```python
from build123d import *

# Parameters (mm, degrees)
PAD_DEPTH       = 20
SKETCH001_W     = 55
SKETCH001_H     = 5
PAD001_DEPTH    = 37
SKETCH002_W     = 8
SKETCH002_H     = 37
PAD002_DEPTH    = 2
SKETCH003_R     = 3.1
POCKET_DEPTH    = 7.001
CHAMFER_SIZE    = 7
FILLET_R        = 2
CHAMFER001_SIZE = 1


with BuildPart() as part:
    # Sketch → Pad (new body)
    with BuildSketch(Plane.XY):
        Polygon((-31.15, 0), (31.15, 0), (31.15, 31.5), (28.15, 31.5), (28.15, 34.5), (34.15, 34.5), (34.15, -3.5), (17.35, -25), (17.35, -33), (-29.15, -33), (-29.15, -11), (-34.15, -3.5), (-34.15, 34.5), (-28.15, 34.5), (-28.15, 31.5), (-31.15, 31.5), align=None)
        Polygon((-21.15, -8), (20.481035, -8), (7.197314, -25), (-21.15, -25), align=None, mode=Mode.SUBTRACT)
    extrude(amount=PAD_DEPTH)

    # Sketch001 (on Face21 of Pad) → Pad001 (join)
    with BuildSketch(Plane(origin=(0, 0, 0), x_dir=(1, 0, 0), z_dir=(0, 0, -1))):
        with Locations((-10.15, 30.5)):
            Rectangle(SKETCH001_W, SKETCH001_H)
    extrude(amount=-PAD001_DEPTH)

    # Sketch002 (on Face25 of Pad001) → Pad002 (join)
    with BuildSketch(Plane.XZ.offset(33)):
        with Locations((4.55, 18.5)):
            Rectangle(SKETCH002_W, SKETCH002_H)
        with Locations((-25.45, 18.5)):
            Rectangle(SKETCH002_W, SKETCH002_H)
    extrude(amount=PAD002_DEPTH)

    # Sketch003 (on Face19 of Pad002) → Pocket (cut, through all)
    with BuildSketch(Plane(origin=(0, -28, 0), x_dir=(-1, 0, 0), z_dir=(0, 1, 0))):
        with Locations((-4.55, 27)):
            Circle(SKETCH003_R)
        with Locations((25.45, 27)):
            Circle(SKETCH003_R)
    extrude(amount=-POCKET_DEPTH, mode=Mode.SUBTRACT)

    # Chamfer
    chamfer_edges = [part.edges().sort_by_distance(p)[0] for p in [
        (-37.65, -30.5, 37),
        (17.35, -30.5, 37),
    ]]
    chamfer(chamfer_edges, length=CHAMFER_SIZE)

    # Fillet
    fillet_edges = [part.edges().sort_by_distance(p)[0] for p in [
        (-29.15, -28, 10),
        (-29.15, -11, 10),
        (-34.15, -3.5, 10),
        (17.35, -25, 10),
        (34.15, -3.5, 10),
        (7.197314, -25, 10),
        (20.481035, -8, 10),
        (-21.15, -8, 10),
        (-21.15, -25, 10),
    ]]
    fillet(fillet_edges, radius=FILLET_R)

    # Chamfer001
    chamfer001_edges = [part.edges().sort_by_distance(p)[0] for p in [
        (-34.15, -28, 33.5),
        (-37.65, -28, 15),
        (-10.15, -28, 37),
        (13.85, -28, 33.5),
        (17.35, -28, 25),
    ]]
    chamfer(chamfer001_edges, length=CHAMFER001_SIZE)


solid = part.part
```
Part model, mm, in its own coordinate system. A direction names the side the tool comes from. Round coordinates to 2 decimals unless told otherwise and drop trailing zeros. Write each loop counter-clockwise with the first axis right and the second up, starting at its lowest first coordinate (ties: lowest second). Pieces come first, ordered by that corner, then holes. Notation, with made-up numbers: (39, 10) -> (89, 10) arc R24 cw to (89, 24) -> close; hole circle Ø3 at (-1.5, 14). An arc over 180 degrees is marked (long way). Return JSON: item names as keys, results as strings. Group by question number.
Q1. Which spindle directions (+Z, -Z, +X, -X, +Y, -Y) get a long thin tool onto all of the face, cutting with end or side? Do faces 4 (the flat face through (-21.45, -34, 18)), 5 (the flat face through (-31.62, -7.295, 9.86)), 6 (the flat face through (-16, -28, 26)). Say none if no direction does.
Q2. Pin check, flat tips, straight feed: pin 1 (1.5 mm diameter, centred on x = 22.5, y = -11.5, fed in from +Z); pin 2 (8 mm diameter, centred on y = -28, z = 19.5, fed in from +X); pin 3 (5 mm diameter, centred on y = -14, z = 21.5, fed in from -X). Stop position of each tip, or through.
Q3. Mould opens along Z. For faces 1 (the cylindrical face through (-27.12, -31.45, 29.61)), 2 (the flat face through (13.9, -30.97, 33.45)), 3 (the flat face through (-31.15, 16, 10)) say: pulls with the +Z half, pulls with the -Z half, needs draft (parallel to the pull), parting line crosses it, or undercut.
Q4. Saw through at B-B on z = 27. Write the cut outline in (x, y), plus the area to 3 significant figures.
Q5. Saw through at C-C on x = 4.55. Write the cut outline in (y, z).
Q6. Saw through at A-A on x = -25.45. Write the cut outline in (y, z), plus the area to 3 significant figures.
Q7. Probe L1, parallel to Y at x = 4, z = 11; L2, parallel to Z at x = 4.55, y = -32.25; L3, parallel to X at y = 14, z = 4.5. List the from-to ranges inside material, lowest first. Write a range as [from, to].
Q8. Saw through at D-D on y = -22. Write the cut outline in (x, z).
Answer:
{
 "1": {"face 4": "+Z, -Z, -Y", "face 5": "+Z, -Z, -X", "face 6": "+Z, -X"},
 "2": {"pin 1": "z = 20", "pin 2": "x = 18.13", "pin 3": "x = -29.15"},
 "3": {"face 1": "undercut", "face 2": "pulls with the +Z half", "face 3": "needs draft"},
 "4": {"outline": "(-37.65, -33) -> (-29.45, -33) -> (-29.45, -35) -> (-28.55, -35) -> (-28.55, -28) -> (-36.65, -28) -> (-37.65, -29) -> close; (-22.35, -35) -> (-21.45, -35) -> (-21.45, -33) -> (0.55, -33) -> (0.55, -35) -> (1.45, -35) -> (1.45, -28) -> (-22.35, -28) -> close; (7.65, -35) -> (8.55, -35) -> (8.55, -33) -> (17.35, -33) -> (17.35, -29) -> (16.35, -28) -> (7.65, -28) -> close", "area": "219 mm2"},
 "5": {"outline": "(-35, 0) -> (-25, 0) -> (-25, 20) -> (-28, 20) -> (-28, 23.9) -> (-35, 23.9) -> close; (-35, 30.1) -> (-28, 30.1) -> (-28, 36) -> (-29, 37) -> (-35, 37) -> close; (-8, 0) -> (0, 0) -> (0, 20) -> (-8, 20) -> close"},
 "6": {"outline": "(-35, 0) -> (0, 0) -> (0, 20) -> (-28, 20) -> (-28, 23.9) -> (-35, 23.9) -> close; (-35, 30.1) -> (-28, 30.1) -> (-28, 36) -> (-29, 37) -> (-35, 37) -> close", "area": "775 mm2"},
 "7": {"L1": "[-35, -25], [-8, 0]", "L2": "[0, 23.9], [30.1, 37]", "L3": "[-34.15, -31.15], [31.15, 34.15]"},
 "8": {"outline": "(-29.15, 0) -> (-21.15, 0) -> (-21.15, 20) -> (-29.15, 20) -> close; (9.54, 0) -> (19.69, 0) -> (19.69, 20) -> (9.54, 20) -> close"}
}
